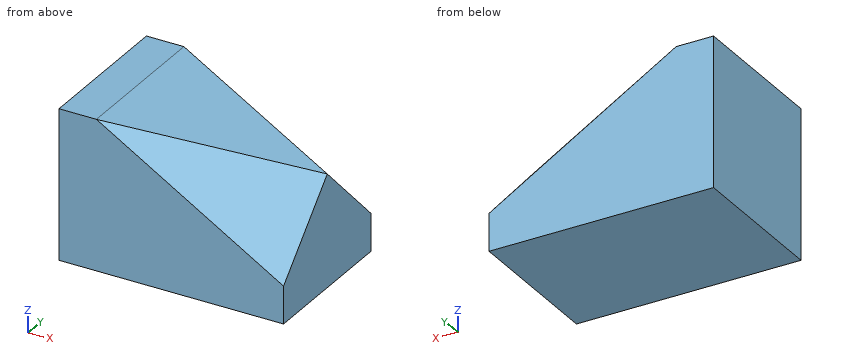
Autodesk Inventor part; units mm, degrees
ref_plane "工作平面3" through (60, 40, 10) normal (-0.3906, -0.6509, -0.6509) x (0, -0.7071, 0.7071)
ref_plane "工作平面4" through (60, 20, 30) normal (-0.3906, 0.6509, -0.6509) x (0, -0.7071, -0.7071)
ref_plane "YZ Plane" through (0, 0, 0) normal (1, 0, 0) x (0, 1, 0)
sketch "草圖1" plane through (0, 0, 0) normal (0, 0, 1) x (1, 0, 0)
  line L0 (0, 0) -> (60, 0)
  line L1 (60, 0) -> (60, 40)
  line L2 (60, 40) -> (0, 40)
  line L3 (0, 40) -> (0, 0)
  dimension "d0" = 60
  dimension "d1" = 40
extrude "擠出1" add sketch "草圖1" along normal blind 40
chamfer "倒角1" distance 50 distance2 10 1 edges at (60, 20, 40) measured on face at (20, 26.6667, 40)
sketch "草圖2" plane through (60, 0, 0) normal (1, 0, 0) x (0, 0, -1)
  line L0 (0, 40) -> (-30, 40)
  line L1 (0, 0) -> (0, 40)
  line L2 (0, 0) -> (-30, 0)
  line L3 (-40, 40) -> (-40, 0)
  point P0 (-10, 40)
  point P1 (-10, 0)
  point P2 (-40, 20)
  dimension "d7" = 10
  dimension "d10" = 10
  dimension "d13" = 20
ref_plane "工作平面3" through (60, 40, 10) normal (-0.3906, -0.6509, -0.6509) x (0, -0.7071, 0.7071)
ref_plane "工作平面4" through (60, 20, 30) normal (-0.3906, 0.6509, -0.6509) x (0, -0.7071, -0.7071)
sketch "草圖5" plane through (60, 40, 10) normal (-0.3906, -0.6509, -0.6509) x (0, -0.7071, 0.7071)
  line L0 (-21.2028, 86.012) -> (46.7944, 86.012)
  line L1 (46.7944, 86.012) -> (46.7944, -28.5442)
  line L2 (46.7944, -28.5442) -> (-21.2028, -28.5442)
  line L3 (-21.2028, -28.5442) -> (-21.2028, 86.012)
  point P0 (21.2132, 41.4259)
extrude "擠出4" cut sketch "草圖5" against normal blind 40
sketch "草圖6" plane through (60, 20, 30) normal (-0.3906, 0.6509, -0.6509) x (0, -0.7071, -0.7071)
  line L0 (-21.2652, 80.224) -> (44.7592, 80.224)
  line L1 (44.7592, 80.224) -> (44.7592, -31.1757)
  line L2 (44.7592, -31.1757) -> (-21.2652, -31.1757)
  line L3 (-21.2652, -31.1757) -> (-21.2652, 80.224)
  point P0 (35.3553, 52.4728)
extrude "擠出5" cut sketch "草圖6" against normal blind 40
Could you check a few things on this model? Use its own coordinates, in mm. Give positions to 0.01 mm unless a question says otherwise; leave off trailing zeros. Write each loop counter-clockwise with the first axis right and the second up, starting at its lowest first coordinate (ties: lowest second). Pieces come first, ordered by that corner, then holes. Notation, with made-up numbers: (-31, -3.75) - (10, -3.75) arc R16 ccw to (10, 21.25) - close; hole circle Ø10 at (24, -29.5). An arc over 180 degrees is marked (long way). One line per item, written item: value. Start each with the question number.
Item 1: Imagine slicing it at B-B, the plane z = 21.5. List the corners of the cut face in (x, y) for me.
Item 2: I'm going to push flat-ended pins straight in: pin 1 (2 mm diameter, centred on x = 31, y = 33.5, fed in from +Z); pin 2 (1.5 mm diameter, centred on x = 24.5, y = 28.5, fed in from +Z); pin 3 (2 mm diameter, centred on y = 29, z = 24, fed in from +X). Where does each tip first touch, or does it pass through?
Item 3: Imagine slicing it at A-A, the plane x = 54. List the corners of the cut face in (y, z) for me.
Item 4: Please list where these lines run through material, in increasing order: line 1 (Y direction, x = 40, z = 22); line 2 (Y direction, x = 46, z = 26.5); line 3 (X direction, y = 34, z = 26). Write a range as from..to.
Geometry says:
1. outline: (0, 0) - (40.83, 0) - (60, 11.5) - (60, 28.5) - (40.83, 40) - (0, 40) - close
2. pin 1: z = 35.07
2. pin 2: z = 37.25
2. pin 3: x = 57.35
3. outline: (0, 0) - (40, 0) - (40, 13.6) - (22.4, 31.2) - (17.6, 31.2) - (0, 13.6) - close
4. line 1: 0..40
4. line 2: 8.1..31.9
4. line 3: 0..43.33
